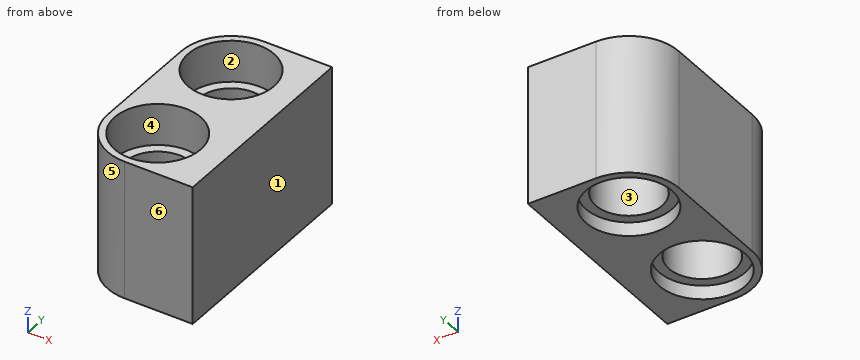
Autodesk Inventor part; units mm, degrees
ref_plane "YZ Plane" through (0, 0, 0) normal (1, 0, 0) x (0, 1, 0)
ref_plane "XZ Plane" through (0, 0, 0) normal (0, 1, 0) x (-1, 0, 0)
ref_plane "XY Plane" through (0, 0, 0) normal (0, 0, 1) x (1, 0, 0)
sketch "Esboço1" plane through (0, 0, 0) normal (0, 0, 1) x (1, 0, 0)
  circle A0 centre (0, 51.501) radius 2.4
  line L0 (4.9, 66.501) -> (4.9, -3.499)
  line L1 (-3.6, 3.501) -> (-3.6, 59.501)
  arc A1 (0, 55.101) -> (-3.6, 51.501) centre (0, 51.501) ccw
  circle A2 centre (0, 43.501) radius 2.4
  arc A3 (-3.6, 43.501) -> (0, 39.901) centre (0, 43.501) ccw
  line L2 (4.9, 55.101) -> (0, 55.101)
  line L3 (0, 55.101) -> (0, 39.901)
  line L4 (0, 39.901) -> (4.9, 39.901)
  line L5 (4.9, 39.901) -> (4.9, 55.101)
  point P0 (0, 0)
extrude "Extrusão1" add sketch "Esboço1" along normal blind 10 contours A0 L3 L2 L0 L4 A2 | A0 L3 A2 A3 L1 A1
sketch "Esboço2" plane through (0, 0, 10) normal (0, 0, 1) x (1, 0, 0)
  circle A0 centre (0, 43.501) radius 3.1
  circle A1 centre (0, 51.501) radius 3.1
  point P0 (0, 0)
extrude "Extrusão2" cut sketch "Esboço2" against normal blind 3
sketch "Esboço3" plane through (0, 0, 0) normal (0, 0, -1) x (-1, 0, 0)
  circle A0 centre (0, 51.501) radius 3.1
  circle A1 centre (0, 51.501) radius 2.4
  circle A2 centre (0, 43.501) radius 3.1
  circle A3 centre (0, 43.501) radius 2.4
  point P0 (0, 0)
extrude "Extrusão3" cut sketch "Esboço3" against normal blind 1 contours A0 | A1 | A2 | A3
properties part number "suporte sensor de cor"
For this review, take the finished solid that the model builds, in its own axes (mm). Face numbers are marked on the shaded views. A direction names the side the tool comes from. Round coordinates to 2 decimals unless told otherwise and drop trailing zeros. Write each loop counter-clockwise with the first axis right and the second up, starting at its lowest first coordinate (ties: lowest second). Pieces come first, ordered by that corner, then holes. Notation, with made-up numbers: M 49.25,-35 L 60.25,-35 A4 ccw 60.25,-29 Z; hole C 67,-21 d6. An arc over 180 degrees is marked long. Write item = value, one per line. Start each with the question number.
(1) Clearance check with flat-ended pins moving along their axes: pin 1 Ø5 at (x, y) = (0, 43.501) entering from +Z; pin 2 Ø5 at (x, y) = (0, 51.501) entering from -Z; pin 3 Ø1.5 at (x, y) = (1.5, 43.5) entering from +Z. State where each tip first meets the part, or that it passes through.
(2) We need section C-C (x = -0.75). Give the boundary of the cut face in (y, z), then the cut area to 3 significant figures.
(3) For the marked faces 1 and 2, list the 3-axis set-ups (+Z, -Z, +X, -X, +Y, -Y) from which the entire face can be reached by the end or side of a thin tool; tool diameter is ignored.
(4) We need section A-A (y = 49.5). Give the boundary of the cut face in (x, z), then the cut area to 3 significant figures.
(5) We need section B-B (z = 8). Give the boundary of the cut face in (x, y).
(6) We need section D-D (y = 52.5). Give the boundary of the cut face in (x, z), then the cut area to 3 significant figures.
(7) For line 1 along Y through (x, z) = (0, 3.5); line 2 along Y through (x, z) = (0, 8.5); line 3 along Z through (x, y) = (1, 48.75), list the stretches that pass through material, from the lowest coordinate up.
(8) The part is to be moulded in two halves that separate along X. For the marked faces 3, 4, 5 and 6, say which applies: +X half, -X half, draft (parallel to the pull), parting line (faces both ways), or undercut.
Results found:
q1.pin_1 = 7
q1.pin_2 = 1
q1.pin_3 = through
q2.outline = M 39.98,0 L 40.49,0 L 40.49,1 L 41.22,1 L 41.22,7 L 40.49,7 L 40.49,10 L 39.98,10 Z; M 45.78,1 L 46.51,1 L 46.51,0 L 48.49,0 L 48.49,1 L 49.22,1 L 49.22,7 L 48.49,7 L 48.49,10 L 46.51,10 L 46.51,7 L 45.78,7 Z; M 53.78,1 L 54.51,1 L 54.51,0 L 55.02,0 L 55.02,10 L 54.51,10 L 54.51,7 L 53.78,7 Z
q2.area = 47.6 mm²
q3.face_1 = +Z, -Z, +X, +Y, -Y
q3.face_2 = +Z
q4.outline = M -3.6,0 L -2.37,0 L -2.37,1 L -1.33,1 L -1.33,7 L -2.37,7 L -2.37,10 L -3.6,10 Z; M 1.33,1 L 2.37,1 L 2.37,0 L 4.9,0 L 4.9,10 L 2.37,10 L 2.37,7 L 1.33,7 Z
q4.area = 50.2 mm²
q5.outline = M -3.6,43.5 A3.6 ccw 0,39.9 L 4.9,39.9 L 4.9,55.1 L 0,55.1 A3.6 ccw -3.6,51.5 Z; hole C 0,43.5 d6.2; hole C 0,51.5 d6.2
q6.outline = M -3.46,0 L -2.93,0 L -2.93,1 L -2.18,1 L -2.18,7 L -2.93,7 L -2.93,10 L -3.46,10 Z; M 2.18,1 L 2.93,1 L 2.93,0 L 4.9,0 L 4.9,10 L 2.93,10 L 2.93,7 L 2.18,7 Z
q6.area = 33.9 mm²
q7.line_1 = 39.9 to 41.1, 45.9 to 49.1, 53.9 to 55.1
q7.line_2 = 39.9 to 40.4, 46.6 to 48.4, 54.6 to 55.1
q7.line_3 = 1 to 7
q8.face_3 = undercut
q8.face_4 = undercut
q8.face_5 = -X half
q8.face_6 = draft
